Study the drawing (mm; zero at the part's minimum x, y, z) and answer. Give positions to 0.01 mm unless a question says otherwise; leave off trailing zeros. Loops run counter-clockwise (first coordinate to the right, second up) from the corner with the lowest first, then second, coordinate; pieces in that order, holes last. Notation, with made-up numbers: (40, -12) - (95, -12) arc R13 cw to (95, 8) - close; hole circle Ø2 at (16.25, -39). An arc over 180 degrees is marked (long way). One line per item, written item: value. Start each with the question number.
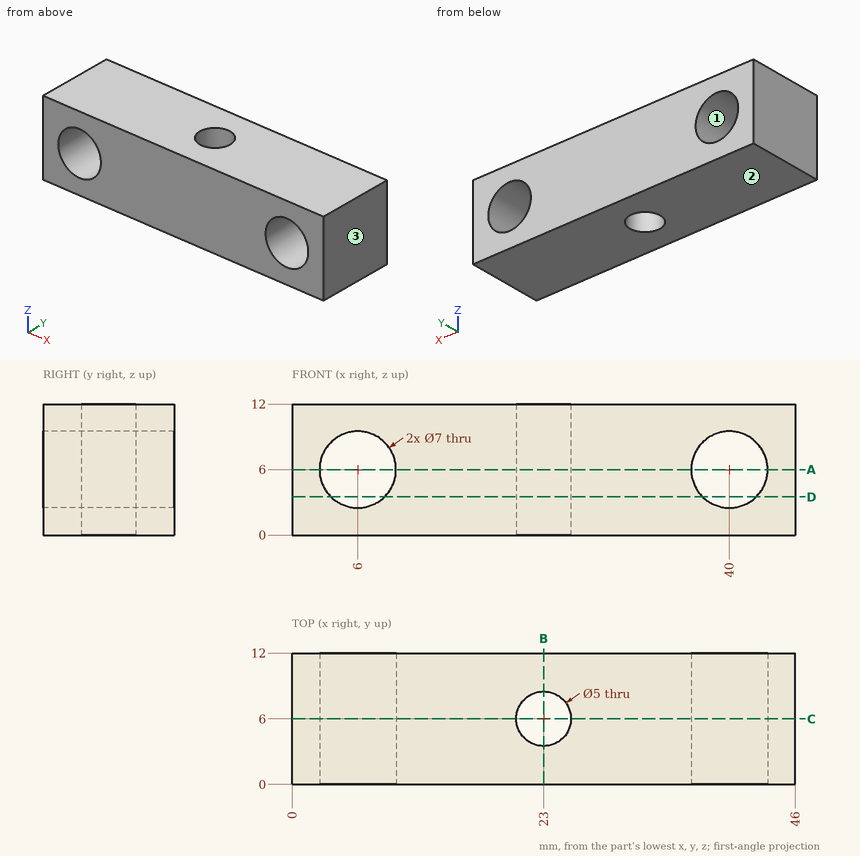
1. A cutting plane is placed at C-C (y = 6). Determine the outline of the cut face in (x, z).
2. Find the intervals of material crossed by L1, parallel to Z at x = 6, y = 8.75; L2, parallel to X at y = 2, z = 9; L3, parallel to X at y = 4.5, z = 6.5, in increasing order. Write a range as [from, to].
3. Determine the mould class of the marked faces 1, 2 and 3 for opening direction Z: released by +Z, released by -Z, zero draft, split by the parting line, or undercut.
4. A cutting plane is placed at D-D (z = 3.5). Determine the outline of the cut face in (x, y).
5. A cutting plane is placed at B-B (x = 23). Determine the outline of the cut face in (y, z), plus the area to 3 significant figures.
6. A cutting plane is placed at A-A (z = 6). Determine the outline of the cut face in (x, y), plus the area to 3 significant figures.
Results below:
1. outline: (0, 0) - (20.5, 0) - (20.5, 12) - (0, 12) - close; (25.5, 0) - (46, 0) - (46, 12) - (25.5, 12) - close; hole circle Ø7 at (6, 6); hole circle Ø7 at (40, 6)
2. L1: z = [0, 2.5], [9.5, 12]
2. L2: x = [0, 4.2], [7.8, 38.2], [41.8, 46]
2. L3: x = [0, 2.54], [9.46, 21], [25, 36.54], [43.46, 46]
3. face 1: undercut
3. face 2: released by -Z
3. face 3: zero draft
4. outline: (0, 0) - (3.55, 0) - (3.55, 12) - (0, 12) - close; (8.45, 0) - (37.55, 0) - (37.55, 12) - (8.45, 12) - close; (42.45, 0) - (46, 0) - (46, 12) - (42.45, 12) - close; hole circle Ø5 at (23, 6)
5. outline: (0, 0) - (3.5, 0) - (3.5, 12) - (0, 12) - close; (8.5, 0) - (12, 0) - (12, 12) - (8.5, 12) - close
5. area: 84.0 mm^2
6. outline: (0, 0) - (2.5, 0) - (2.5, 12) - (0, 12) - close; (9.5, 0) - (36.5, 0) - (36.5, 12) - (9.5, 12) - close; (43.5, 0) - (46, 0) - (46, 12) - (43.5, 12) - close; hole circle Ø5 at (23, 6)
6. area: 364 mm^2
